Source: CAD feature listing. Evaluate the final solid. Frame: model axes, mm. A direction names the side the tool comes from. Coordinates: 2 decimals unless noted, no trailing zeros. Order: outer loops, then holes, each group sorted by start corner. A loop starts at its lowest first (then second) coordinate and runs counter-clockwise, first axis right, second up. Notation, with made-up numbers: (32.5, 5.5) -> (69.5, 5.5) arc R13 cw to (69.5, 15.5) -> close; hole circle Ø10 at (-26, 13). An arc over 180 degrees is marked (long way). Put each result on its own line as item: value.
from build123d import *

# Parameters (mm, degrees)
F0_W     = 25.4
F0_H     = 25.4
F1_DEPTH = 76.2
F2_R     = 7.62
F3_DEPTH = 25.4
F4_W     = 6.35
F4_H     = 25.4
F5_DEPTH = 25.4


with BuildPart() as f1:
    # F0 (on Right) → F1 (new body, symmetric)
    with BuildSketch(Plane.YZ):
        Rectangle(F0_W, F0_H)
    extrude(amount=F1_DEPTH, both=True)

    # F2 (on face) → F3 (cut, through all)
    with BuildSketch(Plane.XZ.offset(12.7)):
        with Locations((63.5, 0)):
            Circle(F2_R)
    extrude(amount=-F3_DEPTH, mode=Mode.SUBTRACT)

    # F4 (on face) → F5 (cut)
    with BuildSketch(Plane.YZ.offset(76.2)):
        Rectangle(F4_W, F4_H)
    extrude(amount=-F5_DEPTH, mode=Mode.SUBTRACT)


solid = f1.part
1. Cut plane C-C on z = 0. Output: boundary loops of the cut face in (x, y) (3 decimals).
Numbers:
outline: (-76.2, -12.7) -> (55.88, -12.7) -> (55.88, -3.175) -> (50.8, -3.175) -> (50.8, 3.175) -> (55.88, 3.175) -> (55.88, 12.7) -> (-76.2, 12.7) -> close; (71.12, -12.7) -> (76.2, -12.7) -> (76.2, -3.175) -> (71.12, -3.175) -> close; (71.12, 3.175) -> (76.2, 3.175) -> (76.2, 12.7) -> (71.12, 12.7) -> close
2. First-contact query: pin 1 (12 mm diameter, centred on x = 63.5, z = 0, fed in from -Y); pin 2 (3 mm diameter, centred on y = 1.5, z = -2, fed in from +X); pin 3 (12.5 mm diameter, centred on x = 67.5, z = 1.5, fed in from -Y). Flat tips, straight axial feed; report the tip coordinate or a pass-through.
Numbers:
pin 1: passes through
pin 2: stops at x = 50.8
pin 3: stops at y = -12.7
3. Cut plane A-A on x = 63.5. Output: boundary loops of the cut face in (y, z) (3 decimals), plus the area to 3 significant figures.
Numbers:
outline: (-12.7, -12.7) -> (-3.175, -12.7) -> (-3.175, -7.62) -> (-12.7, -7.62) -> close; (-12.7, 7.62) -> (-3.175, 7.62) -> (-3.175, 12.7) -> (-12.7, 12.7) -> close; (3.175, -12.7) -> (12.7, -12.7) -> (12.7, -7.62) -> (3.175, -7.62) -> close; (3.175, 7.62) -> (12.7, 7.62) -> (12.7, 12.7) -> (3.175, 12.7) -> close
area: 194 mm2
4. Cut plane D-D on z = -9. Output: boundary loops of the cut face in (x, y) (3 decimals).
Numbers:
outline: (-76.2, -12.7) -> (76.2, -12.7) -> (76.2, -3.175) -> (50.8, -3.175) -> (50.8, 3.175) -> (76.2, 3.175) -> (76.2, 12.7) -> (-76.2, 12.7) -> close
5. Ray query, line 1 along Z through (x, y) = (63.5, 9.5); line 2 along X through (y, z) = (10, -0.5); line 3 along Z through (x, y) = (69, 11.25). Return the intervals inside material, ascending.
Numbers:
line 1: z = -12.7 to -7.62, 7.62 to 12.7
line 2: x = -76.2 to 55.9, 71.1 to 76.2
line 3: z = -12.7 to -5.27, 5.27 to 12.7
6. Set-up query: faces 4 (the flat face through (1, 0, -12.7)), 5 (the flat face through (58, 3.175, 5.5)). Return all of +Z, -Z, +X, -X, +Y, -Y with unobstructed straight access to the full face (end or side cutting, diameter ignored); none if empty.
Numbers:
face 4: -Z, +X, -X, +Y, -Y
face 5: +Z, -Z, +X
7. Pull-direction query (Y, two-part tool) for faces 1 (the flat face through (1, 0, 12.7)), 2 (the flat face through (1, -12.7, 0)), 3 (the flat face through (50.8, 0, 0)); classes: pulls with the +Y half, pulls with the -Y half, needs draft (parallel to the pull), parting line crosses it, or undercut.
Numbers:
face 1: needs draft
face 2: pulls with the -Y half
face 3: undercut
8. Cut plane B-B on y = 5.25. Output: boundary loops of the cut face in (x, z), plus the area to 3 significant figures.
Numbers:
outline: (-76.2, -12.7) -> (76.2, -12.7) -> (76.2, 12.7) -> (-76.2, 12.7) -> close; hole circle Ø15.24 at (63.5, 0)
area: 3,690 mm2
